Part model, mm, in its own coordinate system. A direction names the side the tool comes from. Round coordinates to 2 decimals unless told otherwise and drop trailing zeros. Answer as a JSON object with one key per item and string values. Group by question number.
```python
from build123d import *

# Parameters (mm, degrees)
SKETCH_1_W             = 70
SKETCH_1_H             = 20
SKETCH_1_W_2           = 66
SKETCH_1_H_2           = 16
EXTRUDE_1_DEPTH        = 240
CUT_EXTRUDE_1_REACH    = 22
SKETCH_2_R             = 10
CUT_EXTRUDE_2_REACH    = 22
SKETCH_3_R             = 5
SKETCH_4_R             = 2.1
CUT_EXTRUDE_3_DEPTH    = 21
CUT_EXTRUDE_5_REACH    = 22
CUT_EXTRUDE_8_DEPTH    = 21
SKETCH_13_R            = 3.1
CUT_EXTRUDE_10_DEPTH   = 21
CUT_EXTRUDE_11_REACH   = 22
SKETCH_14_W            = 13
SKETCH_14_H            = 7
FILLET_1_R             = 1
CUT_EXTRUDE_12_REACH   = 22
SKETCH_15_R            = 1
HOLE_WIZARD_M3_1_D     = 2.5
HOLE_WIZARD_M3_1_DEPTH = 20
SKETCH_40_R            = 1.7
CUT_EXTRUDE_21_DEPTH   = 10
SKETCH_49_R            = 4.1
SKETCH_49_R_2          = 2.2
SKETCH_49_R_3          = 5.5
SKETCH_49_R_4          = 3.2
EXTRUDE_2_DEPTH        = 16
SKETCH_50_R            = 1.7
CUT_EXTRUDE_27_DEPTH   = 2
SKETCH_51_W            = 18
SKETCH_51_H            = 65
CUT_EXTRUDE_28_DEPTH   = 2
FILLET_6_R             = 3
CUT_EXTRUDE_29_REACH   = 22
SKETCH_52_R            = 1.3
CUT_EXTRUDE_30_REACH   = 22
SKETCH_53_R            = 1.65


with BuildPart() as part:
    # 草图1 → 凸台-拉伸1 (new body)
    with BuildSketch(Plane.XY):
        Rectangle(SKETCH_1_W, SKETCH_1_H)
        Rectangle(SKETCH_1_W_2, SKETCH_1_H_2, mode=Mode.SUBTRACT)
    extrude(amount=EXTRUDE_1_DEPTH)

    # 草图2 → 切除-拉伸1 (cut, up to next)
    with BuildSketch(Plane(origin=(0, 10, 0), x_dir=(1, 0, 0), z_dir=(0, 1, 0)), mode=Mode.PRIVATE) as cut_extrude_1_sk1:
        with Locations((0, -30)):
            Circle(SKETCH_2_R)
    cut_extrude_1_tool1 = extrude(cut_extrude_1_sk1.sketch, amount=-CUT_EXTRUDE_1_REACH, mode=Mode.PRIVATE) & part.part
    add(cut_extrude_1_tool1.solids().sort_by_distance((0, 10, 30))[0], mode=Mode.SUBTRACT)

    # 草图3 → 切除-拉伸2 (cut, up to next)
    with BuildSketch(Plane(origin=(0, 10, 0), x_dir=(1, 0, 0), z_dir=(0, 1, 0)), mode=Mode.PRIVATE) as cut_extrude_2_sk1:
        with Locations((0, -210)):
            Circle(SKETCH_3_R)
    cut_extrude_2_tool1 = extrude(cut_extrude_2_sk1.sketch, amount=-CUT_EXTRUDE_2_REACH, mode=Mode.PRIVATE) & part.part
    add(cut_extrude_2_tool1.solids().sort_by_distance((0, 10, 210))[0], mode=Mode.SUBTRACT)

    # 草图4 → 切除-拉伸3 (cut, through all)
    with BuildSketch(Plane(origin=(0, 10, 0), x_dir=(1, 0, 0), z_dir=(0, 1, 0))):
        with Locations((-13.980630511, -13.338533362)):
            Circle(SKETCH_4_R)
        with Locations((-21.75, -30)):
            Circle(SKETCH_4_R)
        with Locations((13.980630511, -13.338533362)):
            Circle(SKETCH_4_R)
        with Locations((21.75, -30)):
            Circle(SKETCH_4_R)
        with Locations((13.980630511, -46.661466638)):
            Circle(SKETCH_4_R)
        with Locations((-13.980630511, -46.661466638)):
            Circle(SKETCH_4_R)
    extrude(amount=-CUT_EXTRUDE_3_DEPTH, mode=Mode.SUBTRACT)

    # 草图7 → 切除-拉伸5 (cut, up to next)
    with BuildSketch(Plane.XZ.offset(10), mode=Mode.PRIVATE) as cut_extrude_5_sk1:
        with BuildLine():
            Line((-35, 16.180278489), (-35, 0))
            Line((-35, 0), (-21.308191912, 0))
            ThreePointArc((-21.308191912, 0), (-29.522957546, 6.931803792), (-35, 16.180278489))
        make_face()
    cut_extrude_5_tool1 = extrude(cut_extrude_5_sk1.sketch, amount=-CUT_EXTRUDE_5_REACH, mode=Mode.PRIVATE) & part.part
    add(cut_extrude_5_tool1.solids().sort_by_distance((-30.953915, -10, 4.726426))[0], mode=Mode.SUBTRACT)
    # 草图7 → 切除-拉伸5 (cut, up to next)
    with BuildSketch(Plane.XZ.offset(10), mode=Mode.PRIVATE) as cut_extrude_5_sk2:
        with BuildLine():
            Line((35, 16.180278489), (35, 0))
            Line((35, 0), (21.308191912, 0))
            ThreePointArc((21.308191912, 0), (29.522957546, 6.931803792), (35, 16.180278489))
        make_face()
    cut_extrude_5_tool2 = extrude(cut_extrude_5_sk2.sketch, amount=-CUT_EXTRUDE_5_REACH, mode=Mode.PRIVATE) & part.part
    add(cut_extrude_5_tool2.solids().sort_by_distance((30.953915, -10, 4.726426))[0], mode=Mode.SUBTRACT)

    # 草图10 → 切除-拉伸8 (cut, through all)
    with BuildSketch(Plane(origin=(0, 10, 0), x_dir=(1, 0, 0), z_dir=(0, 1, 0))):
        with BuildLine():
            ThreePointArc((0, -240), (-17.966962187, -237.598213103), (-35, -231.396928288))
            Line((-35, -231.396928288), (-35, -240))
            Line((-35, -240), (0, -240))
        make_face()
        with BuildLine():
            ThreePointArc((35, -231.396928288), (17.966962187, -237.598213103), (0, -240))
            Line((0, -240), (35, -240))
            Line((35, -240), (35, -231.396928288))
        make_face()
    extrude(amount=-CUT_EXTRUDE_8_DEPTH, mode=Mode.SUBTRACT)

    # 草图13 → 切除-拉伸10 (cut, through all)
    with BuildSketch(Plane(origin=(0, 10, 0), x_dir=(1, 0, 0), z_dir=(0, 1, 0))):
        with Locations((-20, -210)):
            Circle(SKETCH_13_R)
        with Locations((-10, -192.679491924)):
            Circle(SKETCH_13_R)
        with Locations((10, -192.679491924)):
            Circle(SKETCH_13_R)
        with Locations((20, -210)):
            Circle(SKETCH_13_R)
        with Locations((10, -227.320508076)):
            Circle(SKETCH_13_R)
        with Locations((-10, -227.320508076)):
            Circle(SKETCH_13_R)
    extrude(amount=-CUT_EXTRUDE_10_DEPTH, mode=Mode.SUBTRACT)

    # 草图14 → 切除-拉伸11 (cut, up to next)
    with BuildSketch(Plane(origin=(0, 10, 0), x_dir=(1, 0, 0), z_dir=(0, 1, 0)), mode=Mode.PRIVATE) as cut_extrude_11_sk1:
        with Locations((0, -186)):
            Rectangle(SKETCH_14_W, SKETCH_14_H)
    cut_extrude_11_tool1 = extrude(cut_extrude_11_sk1.sketch, amount=-CUT_EXTRUDE_11_REACH, mode=Mode.PRIVATE) & part.part
    add(cut_extrude_11_tool1.solids().sort_by_distance((0, 10, 186))[0], mode=Mode.SUBTRACT)

    # 圆角1
    fillet_1_edges = [part.edges().sort_by_distance(p)[0] for p in [
        (-6.5, 9, 189.5),
        (-6.5, 9, 182.5),
        (6.5, 9, 182.5),
        (6.5, 9, 189.5),
    ]]
    fillet(fillet_1_edges, radius=FILLET_1_R)

    # 草图15 → 切除-拉伸12 (cut, up to next)
    with BuildSketch(Plane.XZ.offset(10), mode=Mode.PRIVATE) as cut_extrude_12_sk1:
        with Locations((0, 30)):
            Circle(SKETCH_15_R)
    cut_extrude_12_tool1 = extrude(cut_extrude_12_sk1.sketch, amount=-CUT_EXTRUDE_12_REACH, mode=Mode.PRIVATE) & part.part
    add(cut_extrude_12_tool1.solids().sort_by_distance((0, -10, 30))[0], mode=Mode.SUBTRACT)

    # M3 螺纹孔1
    with Locations(Plane(origin=(0, -10, 30), x_dir=(0, 0, -1), z_dir=(0, -1, 0))):
        with Locations((0, 0), (-180, 0)):
            Hole(HOLE_WIZARD_M3_1_D / 2, depth=HOLE_WIZARD_M3_1_DEPTH)

    # 草图40 → 切除-拉伸21 (cut)
    with BuildSketch(Plane.XZ.offset(10)):
        with Locations((-4, 20)):
            Circle(SKETCH_40_R)
        with Locations((4, 20)):
            Circle(SKETCH_40_R)
    extrude(amount=-CUT_EXTRUDE_21_DEPTH, mode=Mode.SUBTRACT)

    # 草图49 → 凸台-拉伸2 (add)
    with BuildSketch(Plane.XZ.offset(-8)):
        with Locations((-13.980630511, 46.661466638)):
            Circle(SKETCH_49_R)
        with Locations((-13.980630511, 46.661466638)):
            Circle(SKETCH_49_R_2, mode=Mode.SUBTRACT)
        with Locations((-21.75, 30)):
            Circle(SKETCH_49_R)
        with Locations((-21.75, 30)):
            Circle(SKETCH_49_R_2, mode=Mode.SUBTRACT)
        with Locations((-13.980630511, 13.338533362)):
            Circle(SKETCH_49_R)
        with Locations((-13.980630511, 13.338533362)):
            Circle(SKETCH_49_R_2, mode=Mode.SUBTRACT)
        with Locations((13.980630511, 13.338533362)):
            Circle(SKETCH_49_R)
        with Locations((13.980630511, 13.338533362)):
            Circle(SKETCH_49_R_2, mode=Mode.SUBTRACT)
        with Locations((21.75, 30)):
            Circle(SKETCH_49_R)
        with Locations((21.75, 30)):
            Circle(SKETCH_49_R_2, mode=Mode.SUBTRACT)
        with Locations((13.980630511, 46.661466638)):
            Circle(SKETCH_49_R)
        with Locations((13.980630511, 46.661466638)):
            Circle(SKETCH_49_R_2, mode=Mode.SUBTRACT)
        with Locations((-10, 227.320508076)):
            Circle(SKETCH_49_R_3)
        with Locations((-10, 227.320508076)):
            Circle(SKETCH_49_R_4, mode=Mode.SUBTRACT)
        with Locations((10, 227.320508076)):
            Circle(SKETCH_49_R_3)
        with Locations((10, 227.320508076)):
            Circle(SKETCH_49_R_4, mode=Mode.SUBTRACT)
        with Locations((20, 210)):
            Circle(SKETCH_49_R_3)
        with Locations((20, 210)):
            Circle(SKETCH_49_R_4, mode=Mode.SUBTRACT)
        with Locations((10, 192.679491924)):
            Circle(SKETCH_49_R_3)
        with Locations((10, 192.679491924)):
            Circle(SKETCH_49_R_4, mode=Mode.SUBTRACT)
        with Locations((-10, 192.679491924)):
            Circle(SKETCH_49_R_3)
        with Locations((-10, 192.679491924)):
            Circle(SKETCH_49_R_4, mode=Mode.SUBTRACT)
        with Locations((-20, 210)):
            Circle(SKETCH_49_R_3)
        with Locations((-20, 210)):
            Circle(SKETCH_49_R_4, mode=Mode.SUBTRACT)
    extrude(amount=EXTRUDE_2_DEPTH)

    # 草图50 → 切除-拉伸27 (cut)
    with BuildSketch(Plane(origin=(0, 10, 0), x_dir=(1, 0, 0), z_dir=(0, 1, 0))):
        with Locations((-25.75, -93.2)):
            Circle(SKETCH_50_R)
        with Locations((25.75, -93.2)):
            Circle(SKETCH_50_R)
        with Locations((-25.75, -149.8)):
            Circle(SKETCH_50_R)
        with Locations((25.75, -149.8)):
            Circle(SKETCH_50_R)
    extrude(amount=-CUT_EXTRUDE_27_DEPTH, mode=Mode.SUBTRACT)

    # 草图51 → 切除-拉伸28 (cut)
    with BuildSketch(Plane.XZ.offset(10)):
        with Locations((-20, 120.5)):
            Rectangle(SKETCH_51_W, SKETCH_51_H)
    extrude(amount=-CUT_EXTRUDE_28_DEPTH, mode=Mode.SUBTRACT)

    # 圆角6
    fillet_6_edges = [part.edges().sort_by_distance(p)[0] for p in [
        (-11, -9, 153),
        (-11, -9, 88),
        (-29, -9, 88),
        (-29, -9, 153),
    ]]
    fillet(fillet_6_edges, radius=FILLET_6_R)

    # 草图52 → 切除-拉伸29 (cut, up to next)
    with BuildSketch(Plane.XZ.offset(10), mode=Mode.PRIVATE) as cut_extrude_29_sk1:
        with Locations((-24, 168.788603388)):
            Circle(SKETCH_52_R)
    cut_extrude_29_tool1 = extrude(cut_extrude_29_sk1.sketch, amount=-CUT_EXTRUDE_29_REACH, mode=Mode.PRIVATE) & part.part
    add(cut_extrude_29_tool1.solids().sort_by_distance((-24, -10, 168.788603))[0], mode=Mode.SUBTRACT)
    # 草图52 → 切除-拉伸29 (cut, up to next)
    with BuildSketch(Plane.XZ.offset(10), mode=Mode.PRIVATE) as cut_extrude_29_sk2:
        with Locations((-24, 78.788603388)):
            Circle(SKETCH_52_R)
    cut_extrude_29_tool2 = extrude(cut_extrude_29_sk2.sketch, amount=-CUT_EXTRUDE_29_REACH, mode=Mode.PRIVATE) & part.part
    add(cut_extrude_29_tool2.solids().sort_by_distance((-24, -10, 78.788603))[0], mode=Mode.SUBTRACT)
    # 草图52 → 切除-拉伸29 (cut, up to next)
    with BuildSketch(Plane.XZ.offset(10), mode=Mode.PRIVATE) as cut_extrude_29_sk3:
        with Locations((24, 78.788603388)):
            Circle(SKETCH_52_R)
    cut_extrude_29_tool3 = extrude(cut_extrude_29_sk3.sketch, amount=-CUT_EXTRUDE_29_REACH, mode=Mode.PRIVATE) & part.part
    add(cut_extrude_29_tool3.solids().sort_by_distance((24, -10, 78.788603))[0], mode=Mode.SUBTRACT)
    # 草图52 → 切除-拉伸29 (cut, up to next)
    with BuildSketch(Plane.XZ.offset(10), mode=Mode.PRIVATE) as cut_extrude_29_sk4:
        with Locations((24, 168.788603388)):
            Circle(SKETCH_52_R)
    cut_extrude_29_tool4 = extrude(cut_extrude_29_sk4.sketch, amount=-CUT_EXTRUDE_29_REACH, mode=Mode.PRIVATE) & part.part
    add(cut_extrude_29_tool4.solids().sort_by_distance((24, -10, 168.788603))[0], mode=Mode.SUBTRACT)

    # 草图53 → 切除-拉伸30 (cut, up to next)
    with BuildSketch(Plane.XZ.offset(10), mode=Mode.PRIVATE) as cut_extrude_30_sk1:
        with Locations((0, 235.348491094)):
            Circle(SKETCH_53_R)
    cut_extrude_30_tool1 = extrude(cut_extrude_30_sk1.sketch, amount=-CUT_EXTRUDE_30_REACH, mode=Mode.PRIVATE) & part.part
    add(cut_extrude_30_tool1.solids().sort_by_distance((0, -10, 235.348491))[0], mode=Mode.SUBTRACT)


solid = part.part
```
Q1. Two-plate mould, pull along Z, no slides. Class faces 4 (the cylindrical face through (33.453, -0.14, 12.765)), 5 (the cylindrical face through (-2.17, 9.01, 39.76)), 6 (the flat face through (0, -8, 118)), 7 (the flat face through (-35, 0, 122)): +Z half, -Z half, draft (parallel to the pull), parting line (faces both ways), or undercut.
Q2. Which spindle directions (+Z, -Z, +X, -X, +Y, -Y) get a long thin tool onto all of the face, cutting with end or side? Do faces 1 (the cylindrical face through (-10.404, 9.014, 224.247)), 2 (the cylindrical face through (-25.846, 0.112, 30.18)), 3 (the cylindrical face through (-0.651, 9.014, 205.043)). Say none if no direction does.
Q3. Drop flat-ended pins along their axis: pin 1 Ø2 at (x, y) = (-5, 0.5) entering from -Z; pin 2 Ø6 at (x, y) = (-3.5, -2.5) entering from -Z; pin 3 Ø1 at (x, y) = (-13, -6) entering from +Z. Give the stop position or say it passes through.
Q4. Band-saw the part on A-A (y = 4.75). Count the separate pieces of the cut face and the enclosed holes in it, plus the area to 3 significant figures.
Q5. Wall check: line 1 (X direction, y = 9.35, z = 93.2); line 2 (X direction, y = 1.25, z = 205.5); line 3 (X direction, y = 9.5, z = 210). Give the ranges that are in metal, low to high. Write a range as [from, to].
Completed:
{
 "1": {"face 4": "-Z half", "face 5": "undercut", "face 6": "undercut", "face 7": "draft"},
 "2": {"face 1": "+Y, -Y", "face 2": "none", "face 3": "+Y"},
 "3": {"pin 1": "z = 188.9", "pin 2": "z = 188.44", "pin 3": "z = 232.22"},
 "4": {"separate pieces": "14", "enclosed holes": "12", "area": "1,470 mm2"},
 "5": {"line 1": "[-35, -27.45], [-24.05, 24.05], [27.45, 35]", "line 2": "[-35, -33], [-23.16, -16.84], [16.84, 23.16], [33, 35]", "line 3": "[-35, -23.1], [-16.9, -5], [5, 16.9], [23.1, 35]"}
}
